For this review, take the finished solid that the model builds, in its own axes (mm). Face numbers are marked on the shaded views. Give positions to 0.01 mm unless a question says otherwise; leave off trailing zeros. Loops run counter-clockwise (first coordinate to the right, second up) from the corner with the lowest first, then second, coordinate; pieces in that order, holes last.
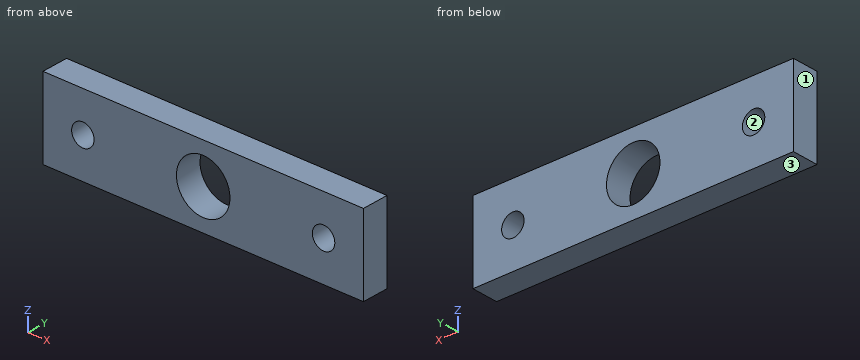
```python
from build123d import *

# Parameters (mm, degrees)
SKETCH1_W           = 76.073
SKETCH1_H           = 19
BOSS_EXTRUDE1_DEPTH = 6.35
CUT_EXTRUDE2_REACH  = 41.716
SKETCH2_R           = 6.35
CUT_EXTRUDE3_REACH  = 41.716
SKETCH4_R           = 2.665


with BuildPart() as part:
    # Sketch1 → Boss-Extrude1 (new body)
    with BuildSketch(Plane(origin=(0, 0, 0), x_dir=(1, 0, 0), z_dir=(0, 1, 0))):
        Rectangle(SKETCH1_W, SKETCH1_H)
    extrude(amount=BOSS_EXTRUDE1_DEPTH)

    # Sketch2 → Cut-Extrude2 (cut, up to next)
    with BuildSketch(Plane(origin=(0, 6.35, 0), x_dir=(1, 0, 0), z_dir=(0, 1, 0)), mode=Mode.PRIVATE) as cut_extrude2_sk1:
        with Locations(Location((0, 0, 0), (0, 0, 270))):
            Circle(SKETCH2_R)
    cut_extrude2_tool1 = extrude(cut_extrude2_sk1.sketch, amount=-CUT_EXTRUDE2_REACH, mode=Mode.PRIVATE) & part.part
    add(cut_extrude2_tool1.solids().sort_by_distance((0, 6.35, 0))[0], mode=Mode.SUBTRACT)

    # Sketch4 → Cut-Extrude3 (cut, up to next)
    with BuildSketch(Plane(origin=(0, 6.35, 0), x_dir=(1, 0, 0), z_dir=(0, 1, 0)), mode=Mode.PRIVATE) as cut_extrude3_sk1:
        with Locations(Location((28.575, 0, 0), (0, 0, 270))):
            Circle(SKETCH4_R)
    cut_extrude3_tool1 = extrude(cut_extrude3_sk1.sketch, amount=-CUT_EXTRUDE3_REACH, mode=Mode.PRIVATE) & part.part
    # Sketch4 → Cut-Extrude3 (cut, up to next)
    with BuildSketch(Plane(origin=(0, 6.35, 0), x_dir=(1, 0, 0), z_dir=(0, 1, 0)), mode=Mode.PRIVATE) as cut_extrude3_sk2:
        with Locations(Location((-28.575, 0, 0), (0, 0, 90))):
            Circle(SKETCH4_R)
    cut_extrude3_tool2 = extrude(cut_extrude3_sk2.sketch, amount=-CUT_EXTRUDE3_REACH, mode=Mode.PRIVATE) & part.part
    add(cut_extrude3_tool1.solids().sort_by_distance((28.575, 6.35, 0))[0], mode=Mode.SUBTRACT)
    add(cut_extrude3_tool2.solids().sort_by_distance((-28.575, 6.35, 0))[0], mode=Mode.SUBTRACT)


solid = part.part
```
Item 1: The part is to be moulded in two halves that separate along X. For the marked faces 1, 2 and 3, say which applies: released by +X, released by -X, zero draft, split by the parting line, or undercut.
Answer:
face 1: released by -X
face 2: undercut
face 3: zero draft
Item 2: For L1, parallel to X at y = 1.75, z = 0; L2, parallel to X at y = 2.75, z = 3.75; L3, parallel to X at y = 4.25, z = 5.5, list the stretches that pass through material, from the lowest coordinate up.
Answer:
L1: x = -38.04 to -31.24, -25.91 to -6.35, 6.35 to 25.91, 31.24 to 38.04
L2: x = -38.04 to -5.12, 5.12 to 38.04
L3: x = -38.04 to -3.17, 3.17 to 38.04
Item 3: Take a section at B-B on z = 0. Give the boundary of the cut face in (x, y).
Answer:
outline: (-38.04, 0) - (-31.24, 0) - (-31.24, 6.35) - (-38.04, 6.35) - close; (-25.91, 0) - (-6.35, 0) - (-6.35, 6.35) - (-25.91, 6.35) - close; (6.35, 0) - (25.91, 0) - (25.91, 6.35) - (6.35, 6.35) - close; (31.24, 0) - (38.04, 0) - (38.04, 6.35) - (31.24, 6.35) - close
Item 4: Take a section at C-C on z = 3.75. Give the boundary of the cut face in (x, y), and give its area (3 significant figures).
Answer:
outline: (-38.04, 0) - (-5.12, 0) - (-5.12, 6.35) - (-38.04, 6.35) - close; (5.12, 0) - (38.04, 0) - (38.04, 6.35) - (5.12, 6.35) - close
area: 418 mm2
Item 5: Take a section at A-A on x = 0. Give the boundary of the cut face in (y, z).
Answer:
outline: (0, -9.5) - (6.35, -9.5) - (6.35, -6.35) - (0, -6.35) - close; (0, 6.35) - (6.35, 6.35) - (6.35, 9.5) - (0, 9.5) - close
Item 6: Clearance check with a flat-ended pin moving along its axis: pin 1 Ø6 at (x, z) = (28.575, 0) entering from -Y. State where the tip first meets the part, or that it passes through.
Answer:
pin 1: stops at y = 0
Item 7: Take a section at D-D on y = 2.75. State how many separate pieces and enclosed holes the cut face has, and give its area (3 significant figures).
Answer:
separate pieces: 1
enclosed holes: 3
area: 1,270 mm2
